Read the model definition and answer for the solid it produces. Units are mm, in the model's axes. A direction names the side the tool comes from. Coordinates: 2 decimals unless noted, no trailing zeros. Write each loop counter-clockwise with the first axis right and the second up, starting at its lowest first coordinate (ties: lowest second). Pieces come first, ordered by that corner, then holes.
1) Which of the six approach directions +Z, -Z, +X, -X, +Y, -Y give full straight-line access (tool end or side, diameter ignored) to faces 1 (the face through (-73.866, -14, 7)), 2 (the face through (-78, -7, 7)), 3 (the face through (-76.5, -9, 8)), 4 (the face through (-73.866, 14, 7))?
2) The part is cut by section B-B (x = 46.5). Determine the outline of the cut face in (y, z).
3) The part is cut by section A-A (z = 7.25). Determine the outline of the cut face in (x, y), then the cut area to 3 significant figures.
4) Each of these flat-tipped pins is pushed along its axis until it touches: pin 1 Ø6 at (x, z) = (32, 1.5) entering from +Y; pin 2 Ø1.5 at (x, y) = (-56, -9) entering from -Z; pin 3 Ø1.5 at (x, z) = (-56.5, 2) entering from -Y; pin 4 Ø5.5 at (x, y) = (26.5, 0) entering from +Z. Where does it stop, or does it pass through?
5) The part is cut by section C-C (y = 0). Give the number of separate pieces and of enclosed holes in the cut face, then the cut area to 3 significant figures.
6) Determine the mould class of faces 5 (the face through (79.478, -1, 7)), 6 (the face through (-78, 7, 7)), 7 (the face through (73.866, 13, 7)) for opening direction X: +X half, -X half, draft (parallel to the pull), parting line (faces both ways), or undercut.
7) Find the intervals of material crossed by line 1 (Y direction, x = 46.5, z = 1.05); line 2 (X direction, y = -11, z = 1.25); line 3 (X direction, y = -10.25, z = 6), in increasing order.
from build123d import *

# Parameters (mm, degrees)
SKETCH1_W                = 153
SKETCH1_H                = 24
BOSS_EXTRUDE1_DEPTH      = 3
BOSS_EXTRUDE2_DEPTH      = 10
BOSS_EXTRUDE2_DEPTH_BACK = 3
CUT_EXTRUDE1_DEPTH       = 3.977609852
CUT_EXTRUDE1_DEPTH_BACK  = 27.977609852
CUT_EXTRUDE2_START       = -4
SKETCH5_R                = 1.75
CUT_EXTRUDE2_DEPTH       = 15
FILLET1_R                = 2
LPATTERN1_COUNT          = 8
LPATTERN1_PITCH          = 20


with BuildPart() as part:
    # Sketch1 → Boss-Extrude1 (new body)
    with BuildSketch(Plane.XY):
        Rectangle(SKETCH1_W, SKETCH1_H)
    extrude(amount=BOSS_EXTRUDE1_DEPTH)

    # Sketch3 → Boss-Extrude2 (add, two sides)
    with BuildSketch(Plane.XY.offset(3)) as boss_extrude2_sk:
        Polygon((-79.477609852, -9.365840911), (-79.477609852, -12.365840911), (-79.477609852, -14.977609852), (-76.865840911, -14.977609852), (-73.865840911, -14.977609852), (-73.865840911, -12), (-76.5, -12), (-76.5, -9.365840911), (-76.5, -7), (-79.477609852, -7), align=None)
        Polygon((-73.865840911, 14.977609852), (-73.865840911, 12), (-76.5, 12), (-76.5, 9.365840911), (-76.5, 7), (-79.477609852, 7), (-79.477609852, 9.365840911), (-79.477609852, 12.365840911), (-79.477609852, 14.977609852), (-76.865840911, 14.977609852), align=None)
        Polygon((79.477609852, 9.365840911), (79.477609852, -9.365840911), (79.477609852, -12.365840911), (79.477609852, -14.977609852), (76.865840911, -14.977609852), (73.865840911, -14.977609852), (73.865840911, -12), (76.5, -12), (76.5, -9.365840911), (76.5, 9.365840911), (76.5, 12), (73.865840911, 12), (73.865840911, 14.977609852), (76.865840911, 14.977609852), (79.477609852, 14.977609852), (79.477609852, 12.365840911), align=None)
    extrude(amount=BOSS_EXTRUDE2_DEPTH)
    extrude(boss_extrude2_sk.sketch, amount=-BOSS_EXTRUDE2_DEPTH_BACK)

    # Sketch4 → Cut-Extrude1 (cut, two sides)
    with BuildSketch(Plane.XZ.offset(12)) as cut_extrude1_sk:
        Polygon((-12.954, 2), (-12.954, 0), (12.954, 0), (12.954, 2), (0, 2.06825053), align=None)
    extrude(amount=CUT_EXTRUDE1_DEPTH, mode=Mode.SUBTRACT)
    extrude(cut_extrude1_sk.sketch, amount=-CUT_EXTRUDE1_DEPTH_BACK, mode=Mode.SUBTRACT)

    # Sketch5 → Cut-Extrude2 (cut)
    with BuildSketch(Plane.XY.offset(3).offset(CUT_EXTRUDE2_START)):
        with Locations((-73.5, 0)):
            Circle(SKETCH5_R)
    cut_extrude2 = extrude(amount=CUT_EXTRUDE2_DEPTH, mode=Mode.SUBTRACT)

    # Fillet1
    fillet1_edges = [part.edges().sort_by_distance(p)[0] for p in [
        (-76.5, 12, 8),
        (-76.5, -12, 8),
        (76.5, -12, 8),
        (79.477609852, 14.977609852, 6.5),
    ]]
    fillet(fillet1_edges, radius=FILLET1_R)

    # LPattern1: Cut-Extrude2 ×8, 1 skipped
    with Locations(*[(i * LPATTERN1_PITCH, 0, 0) for i in range(1, LPATTERN1_COUNT) if i not in (4,)]):
        add(cut_extrude2, mode=Mode.SUBTRACT)


solid = part.part
Reported:
1. face 1: +Z, -Z, -Y
1. face 2: +Z, -Z, -X
1. face 3: +Z
1. face 4: +Z, -Z, +Y
2. outline: (-12, 0) - (-1.75, 0) - (-1.75, 3) - (-12, 3) - close; (1.75, 0) - (12, 0) - (12, 3) - (1.75, 3) - close
3. outline: (-79.48, -14.98) - (-73.87, -14.98) - (-73.87, -12) - (-74.5, -12) arc R2 cw to (-76.5, -10) - (-76.5, -7) - (-79.48, -7) - close; (-79.48, 7) - (-76.5, 7) - (-76.5, 10) arc R2 cw to (-74.5, 12) - (-73.87, 12) - (-73.87, 14.98) - (-79.48, 14.98) - close; (73.87, -14.98) - (79.48, -14.98) - (79.48, 12.98) arc R2 ccw to (77.48, 14.98) - (73.87, 14.98) - (73.87, 12) - (76.5, 12) - (76.5, -10) arc R2 cw to (74.5, -12) - (73.87, -12) - close
3. area: 170 mm2
4. pin 1: stops at y = 12
4. pin 2: stops at z = 0
4. pin 3: stops at y = -12
4. pin 4: stops at z = 3
5. separate pieces: 8
5. enclosed holes: 0
5. area: 374 mm2
6. face 5: +X half
6. face 6: draft
6. face 7: undercut
7. line 1: y = -12 to -1.75, 1.75 to 12
7. line 2: x = -79.48 to -12.95, 12.95 to 79.48
7. line 3: x = -79.48 to -76.48, 76.48 to 79.48
